CAD build for the part. Positions are in the model's coordinates, mm. Face numbers are marked on the shaded views. A direction names the side the tool comes from. Give positions to 0.01 mm unless a question says otherwise; leave off trailing zeros. Order: outer loops, then holes, each group sorted by start corner. A loop starts at its lowest first (then second) coordinate and runs counter-clockwise, first axis right, second up.
Item 1: Band-saw the part on A-A on x = 34. Give the cut face in (y, z), plus the area to 3 significant figures.
Item 2: Two-plate mould, pull along X, no slides. Class the marked faces 1, 2 and 3: released by +X, released by -X, zero draft, split by the parting line, or undercut.
Item 3: Band-saw the part on B-B on y = 0. Count the separate pieces of the cut face and the enclosed holes in it, plus the area to 3 significant figures.
Item 4: Which spindle directions (+Z, -Z, +X, -X, +Y, -Y) get a long thin tool onto all of the face, cutting with end or side? Do the marked faces 4 and 5. Say none if no direction does.
Item 5: Wall check: L1, parallel to Y at x = 43, z = 0; L2, parallel to Y at x = 86.5, z = 12.5; L3, parallel to Z at x = 33.5, y = 5.5. Give the ranges that are in metal, low to high.
Item 6: Band-saw the part on D-D on x = 106.5. Give the cut face in (y, z).
Item 7: Flat gauge pins, fed straight in: P1, Ø8, axis at y = 0, z = 51.63, coming from the +X side (3 decimals); P2, Ø12, axis at x = 103.5, y = 5.5, coming from the -Z side; P3, Ø8, axis at x = 19, z = -6, coming from the +Y side; P4, Ø4, axis at y = 0, z = -51.63, coming from the -X side. Where does each tip first touch, or does it go through?
```python
from build123d import *

# Parameters (mm, degrees)
FLANGE_HOLES_D     = 5.1054
DOWEL_HOLES_D      = 4.7625
DOWEL_HOLES_DEPTH  = 6.35
DOWEL_HOLES_TIP    = 1.430799349
FILLET1_R          = 8.89
CHAMFER1_SIZE      = 2.141545552
CHAMFER1_SIZE_2    = 2.54
SKETCH14_R         = 46.2915
SKETCH14_R_2       = 40.9575
CUT_EXTRUDE1_DEPTH = 2.3876


with BuildPart() as part:
    # Sketch2 → Main Structure (revolve)
    with BuildSketch(Plane.XY, mode=Mode.PRIVATE) as main_structure_sk:
        Polygon((0, 20.583496156), (0, 56.35625), (9.525, 56.35625), (9.525, 16.256), (66.806461084, 16.256), (139.7, 31.75), (139.7, 29.592458901), (60.325, 12.720781818), (60.325, 14.351), (10.795, 14.351), align=None)
    revolve(main_structure_sk.sketch.rotate(Axis((0, 0, 0), (1, 0, 0)), 90), axis=Axis((0, 0, 0), (1, 0, 0)))

    # Flange Holes (through all)
    with Locations(Plane.ZY):
        with Locations((0, -51.6255), (-25.81275, -44.708994483), (-44.708994483, -25.81275), (-51.6255, 0), (-44.708994483, 25.81275), (-25.81275, 44.708994483), (0, 51.6255), (25.81275, 44.708994483), (44.708994483, 25.81275), (51.6255, 0), (44.708994483, -25.81275), (25.81275, -44.708994483)):
            Hole(FLANGE_HOLES_D / 2)

    # Dowel Holes
    with Locations(Plane.ZY):
        with Locations((49.866403745, -13.361662613), (-49.866403745, 13.361662613)):
            Hole(DOWEL_HOLES_D / 2, depth=DOWEL_HOLES_DEPTH)
            with Locations((0, 0, -(DOWEL_HOLES_DEPTH + DOWEL_HOLES_TIP / 2))):  # 118° drill point
                Cone(0, DOWEL_HOLES_D / 2, DOWEL_HOLES_TIP, mode=Mode.SUBTRACT)

    # Fillet1
    fillet1_edges = [part.edges().sort_by_distance(p)[0] for p in [
        (9.525, 0, -16.256),
    ]]
    fillet(fillet1_edges, radius=FILLET1_R)

    # Sketch13 → Cut-Revolve1 (revolve, cut)
    with BuildSketch(Plane(origin=(0, 0, 0), x_dir=(1, 0, 0), z_dir=(0, 1, 0)), mode=Mode.PRIVATE) as cut_revolve1_sk:
        Polygon((0, 36), (3.149591887, 0), (0, 0), align=None)
    revolve(cut_revolve1_sk.sketch.rotate(Axis((3.149591887, 0, 0), (-1, 0, 0)), 180), axis=Axis((3.149591887, 0, 0), (-1, 0, 0)), mode=Mode.SUBTRACT)

    # Chamfer1
    # the kernel refuses this chamfer: 2.54, 2.141545552 mm, written as the material it takes off along each edge
    with BuildSketch(Plane(origin=(139.7, 0, 0), x_dir=(0, 0, 1), z_dir=(0, 1, 0))) as chamfer1_piece_1:
        Polygon((31.75 - CHAMFER1_SIZE * 0.207911690799, -CHAMFER1_SIZE * 0.978147600645), (31.75 - CHAMFER1_SIZE_2, 0), (31.75, 0), align=None)
    revolve(axis=Axis((139.7, 0, 0), (1, 0, 0)), mode=Mode.SUBTRACT)

    # Sketch14 → Cut-Extrude1 (cut)
    with BuildSketch(Plane.ZY):
        Circle(SKETCH14_R)
        Circle(SKETCH14_R_2, mode=Mode.SUBTRACT)
    extrude(amount=-CUT_EXTRUDE1_DEPTH, mode=Mode.SUBTRACT)


solid = part.part
```
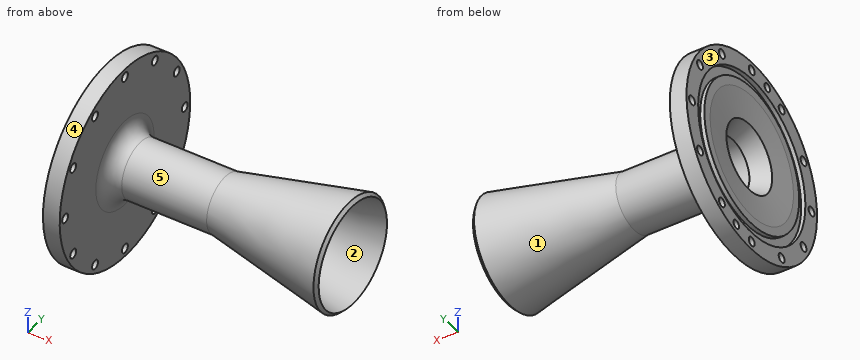
The answers:
1. outline: circle Ø32.51 at (0, 0); hole circle Ø28.7 at (0, 0)
1. area: 183 mm2
2. face 1: undercut
2. face 2: released by +X
2. face 3: released by -X
3. separate pieces: 4
3. enclosed holes: 0
3. area: 1,160 mm2
4. face 4: +X, -X
4. face 5: none
5. L1: y = -16.26 to -14.35, 14.35 to 16.26
5. L2: y = -16.17 to -13.34, 13.34 to 16.17
5. L3: z = -15.3 to -13.26, 13.26 to 15.3
6. outline: circle Ø49.39 at (0, 0); hole circle Ø45.07 at (0, 0)
7. P1: stops at x = 9.525
7. P2: stops at z = -25.04
7. P3: stops at y = 16.26
7. P4: passes through
